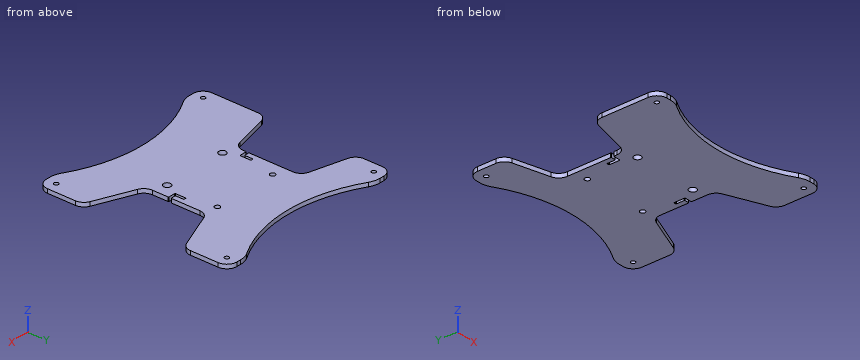
from build123d import *

# Parameters (mm, degrees)
SKETCH1_R           = 2.1
SKETCH1_R_2         = 2.55
SKETCH1_R_3         = 3.6
BOSS_EXTRUDE1_DEPTH = 4


with BuildPart() as part:
    # Sketch1 → Boss-Extrude1 (new body)
    with BuildSketch(Plane(origin=(0, 0, 0), x_dir=(-1, 0, 0), z_dir=(0, 0, -1))):
        with BuildLine():
            Line((87.42535625, -29.106339063), (52.57464375, -20.393660937))
            ThreePointArc((52.57464375, -20.393660937), (47.11794562, -16.84635803), (45, -10.692235936))
            Line((45, -10.692235936), (45, -8))
            ThreePointArc((45, -8), (44.853553391, -7.646446609), (44.5, -7.5))
            Line((44.5, -7.5), (38, -7.5))
            ThreePointArc((38, -7.5), (37.646446609, -7.353553391), (37.5, -7))
            Line((37.5, -7), (37.5, 3))
            ThreePointArc((37.5, 3), (37.646446609, 3.353553391), (38, 3.5))
            Line((38, 3.5), (39.5, 3.5))
            ThreePointArc((39.5, 3.5), (39.853553391, 3.353553391), (40, 3))
            Line((40, 3), (40, -4.5))
            ThreePointArc((40, -4.5), (40.146446609, -4.853553391), (40.5, -5))
            Line((40.5, -5), (44.5, -5))
            ThreePointArc((44.5, -5), (44.853553391, -4.853553391), (45, -4.5))
            Line((45, -4.5), (45, 38.692235936))
            ThreePointArc((45, 38.692235936), (47.11794562, 44.84635803), (52.57464375, 48.393660937))
            Line((52.57464375, 48.393660937), (87.42535625, 57.106339063))
            ThreePointArc((87.42535625, 57.106339063), (92.88205438, 60.65364197), (95, 66.807764064))
            Line((95, 66.807764064), (95, 85))
            ThreePointArc((95, 85), (92.071067812, 92.071067812), (85, 95))
            Line((85, 95), (80.600023778, 95))
            ThreePointArc((80.600023778, 95), (75.38177505, 94.307249421), (70.525020806, 92.276988022))
            ThreePointArc((70.525020806, 92.276988022), (0, 73.215904175), (-70.525020806, 92.276988022))
            ThreePointArc((-70.525020806, 92.276988022), (-75.38177505, 94.307249421), (-80.600023778, 95))
            Line((-80.600023778, 95), (-85, 95))
            ThreePointArc((-85, 95), (-92.071067812, 92.071067812), (-95, 85))
            Line((-95, 85), (-95, 57.30993956))
            ThreePointArc((-95, 57.30993956), (-93.292887614, 51.721736358), (-88.754396995, 48.041471336))
            Line((-88.754396995, 48.041471336), (-51.245603005, 32.847708996))
            ThreePointArc((-51.245603005, 32.847708996), (-46.707112386, 29.167443975), (-45, 23.579240773))
            Line((-45, 23.579240773), (-45, -4.5))
            ThreePointArc((-45, -4.5), (-44.853553391, -4.853553391), (-44.5, -5))
            Line((-44.5, -5), (-40.5, -5))
            ThreePointArc((-40.5, -5), (-40.146446609, -4.853553391), (-40, -4.5))
            Line((-40, -4.5), (-40, 3))
            ThreePointArc((-40, 3), (-39.853553391, 3.353553391), (-39.5, 3.5))
            Line((-39.5, 3.5), (-38, 3.5))
            ThreePointArc((-38, 3.5), (-37.646446609, 3.353553391), (-37.5, 3))
            Line((-37.5, 3), (-37.5, -7))
            ThreePointArc((-37.5, -7), (-37.646446609, -7.353553391), (-38, -7.5))
            Line((-38, -7.5), (-44.5, -7.5))
            ThreePointArc((-44.5, -7.5), (-44.853553391, -7.646446609), (-45, -8))
            Line((-45, -8), (-45, -23.579240773))
            ThreePointArc((-45, -23.579240773), (-46.707112386, -29.167443975), (-51.245603005, -32.847708996))
            Line((-51.245603005, -32.847708996), (-88.754396995, -48.041471336))
            ThreePointArc((-88.754396995, -48.041471336), (-93.292887614, -51.721736358), (-95, -57.30993956))
            Line((-95, -57.30993956), (-95, -85))
            ThreePointArc((-95, -85), (-92.071067812, -92.071067812), (-85, -95))
            Line((-85, -95), (-80.600023778, -95))
            ThreePointArc((-80.600023778, -95), (-75.38177505, -94.307249421), (-70.525020806, -92.276988022))
            ThreePointArc((-70.525020806, -92.276988022), (0, -73.215904175), (70.525020806, -92.276988022))
            ThreePointArc((70.525020806, -92.276988022), (75.38177505, -94.307249421), (80.600023778, -95))
            Line((80.600023778, -95), (85, -95))
            ThreePointArc((85, -95), (92.071067812, -92.071067812), (95, -85))
            Line((95, -85), (95, -38.807764064))
            ThreePointArc((95, -38.807764064), (92.88205438, -32.65364197), (87.42535625, -29.106339063))
        make_face()
        with Locations((-85, -85)):
            Circle(SKETCH1_R, mode=Mode.SUBTRACT)
        with Locations((-85, 85)):
            Circle(SKETCH1_R, mode=Mode.SUBTRACT)
        with Locations((85, 85)):
            Circle(SKETCH1_R, mode=Mode.SUBTRACT)
        with Locations((85, -85)):
            Circle(SKETCH1_R, mode=Mode.SUBTRACT)
        with Locations((32, 29.9)):
            Circle(SKETCH1_R_2, mode=Mode.SUBTRACT)
        with Locations((32, -20.1)):
            Circle(SKETCH1_R_3, mode=Mode.SUBTRACT)
        with Locations((-32, -20.1)):
            Circle(SKETCH1_R_3, mode=Mode.SUBTRACT)
        with Locations((-32, 29.9)):
            Circle(SKETCH1_R_2, mode=Mode.SUBTRACT)
    extrude(amount=-BOSS_EXTRUDE1_DEPTH)


solid = part.part
Could you check a few things on this model? Use its own coordinates, in mm. Give positions to 0.01 mm unless a question says otherwise; leave off trailing zeros. Write each loop counter-clockwise with the first axis right and the second up, starting at its lowest first coordinate (ties: lowest second). Pieces come first, ordered by that corner, then holes. Notation, with made-up numbers: (31.25, 82.5) - (76.25, 82.5) arc R16 ccw to (76.25, 88.5) - close; hole circle Ø4 at (85.25, -16). An arc over 180 degrees is marked (long way). Use CSV: the item, a comma, the result in double quotes. Start each with the question number.
Item 1: I want a section at D-D, the plane x = -21. Please give me the cut outline in (y, z).
Item 2: I want a section at B-B, the plane z = 1. Give the number of separate pieces and of enclosed holes in the cut face, then the cut area to 3 significant figures.
Item 3: I want a section at A-A, the plane x = 32. Please give me the cut outline in (y, z).
Item 4: If I drill on line 1 along Y through (x, z) = (32, 1.95); line 2 along Y through (x, z) = (85.5, 0.9); line 3 along Y through (x, z) = (85, 1.85), over which ranges is the centre line in solid material (lowest first)?
Item 5: I'm going to push flat-ended pins straight in: pin 1 (1 mm diameter, centred on y = -8.5, z = 3.5, fed in from +X); pin 2 (1.5 mm diameter, centred on x = 38.5, z = 1.5, fed in from -Y); pin 3 (2 mm diameter, centred on x = 42, z = 1.5, fed in from -Y). Where does each tip first touch, or does it pass through?
Item 6: I want a section at C-C, the plane x = 3.5. Please give me the cut outline in (y, z).
Findings:
1,outline,"(-74.8, 0) - (74.8, 0) - (74.8, 4) - (-74.8, 4) - close"
2,separate pieces,"1"
2,enclosed holes,"8"
2,area,"23,400 mm2"
3,outline,"(-76.92, 0) - (-23.7, 0) - (-23.7, 4) - (-76.92, 4) - close; (-16.5, 0) - (27.35, 0) - (27.35, 4) - (-16.5, 4) - close; (32.45, 0) - (76.92, 0) - (76.92, 4) - (32.45, 4) - close"
4,line 1,"y = -76.92 to -23.7, -16.5 to 27.35, 32.45 to 76.92"
4,line 2,"y = -94.99 to -87.04, -82.96 to -46.72, 46.72 to 82.96, 87.04 to 94.99"
4,line 3,"y = -95 to -87.1, -82.9 to -46.52, 46.52 to 82.9, 87.1 to 95"
5,pin 1,"stops at x = 45"
5,pin 2,"stops at y = -78.83"
5,pin 3,"stops at y = -79.98"
6,outline,"(-73.26, 0) - (73.26, 0) - (73.26, 4) - (-73.26, 4) - close"
